from build123d import *

# Parameters (mm, degrees)
F1_DEPTH = 140


with BuildPart() as f1:
    # F0 (on Right) → F1 (new body)
    with BuildSketch(Plane.YZ):
        Polygon((3, 0), (0, 0), (-6, 0), (-4.8, -1.2), (38, -1.2), (38, 0), align=None)
        Polygon((3, 32), (3, 0), (38, 0), (38, 37), (3, 37), align=None)
        Polygon((2.247623, 32), (3, 32), (3, 37), (2.422227, 37), align=None)
        Polygon((1.2, 2), (2.247623, 32), (2.422227, 37), (1.222227, 37), (0, 2), align=None)
    extrude(amount=F1_DEPTH)


solid = f1.part
Part model, mm, in its own coordinate system. A direction names the side the tool comes from. Give positions to 0.01 mm unless a question says otherwise; leave off trailing zeros. Loops run counter-clockwise (first coordinate to the right, second up) from the corner with the lowest first, then second, coordinate; pieces in that order, holes last. Notation, with made-up numbers: M -31.75,2 L 2.25,2 A14 ccw 2.25,20 Z; hole C 39.25,89 d3. An arc over 180 degrees is marked long. Put each result on its own line as item: value. Start each with the question number.
1) 3-axis set-ups, long thin cutter, end or side, ignore diameter. For faces 1 (the flat face through (69, -1, 0)), 2 (the flat face through (69, 16, -1.2)): which of +Z, -Z, +X, -X, +Y, -Y reach the whole face in a straight line?
2) Flat gauge pins, fed straight in: pin 1 (8 mm diameter, centred on y = 12, z = 8.5, fed in from -X); pin 2 (2.5 mm diameter, centred on x = 36.5, y = -2.5, fed in from +Z). Where does each tip first touch, or does it go through?
3) Saw through at A-A (x = 9.5). List the corners of the cut face in (y, z), then the cut area to 3 significant figures.
4) Probe probe 1 along Z at (x, y) = (46, -3); probe 2 along Y at (x, z) = (49, 1.5); probe 3 along Y at (x, z) = (94.5, 18). List the from-to ranges inside material, lowest first.
5) Saw through at B-B (z = 11.5). List the corners of the cut face in (x, y).
6) Pull direction Z, two halves, no side cores. Call faces 3 (the flat face through (0, 21, 18)), 4 (the flat face through (69, 3, 16)), 5 (the flat face through (69, 20, 37)): +Z half, -Z half, draft (parallel to the pull), parting line (faces both ways), or undercut.
Numbers:
1. face 1: +X, -X, -Y
1. face 2: -Z, +X, -X, +Y, -Y
2. pin 1: x = 0
2. pin 2: z = 0
3. outline: M -6,0 L -4.8,-1.2 L 38,-1.2 L 38,37 L 1.22,37 L 0,2 L 1.2,2 L 2.25,32 L 3,32 L 3,0 Z
3. area: 1,390 mm^2
4. probe 1: -1.2 to 0
4. probe 2: 3 to 38
4. probe 3: 0.56 to 1.76, 3 to 38
5. outline: M 0,0.33 L 140,0.33 L 140,1.53 L 0,1.53 Z; M 0,3 L 140,3 L 140,38 L 0,38 Z
6. face 3: draft
6. face 4: undercut
6. face 5: +Z half
